For this review, take the finished solid that the model builds, in its own axes (mm). Coordinates: 2 decimals unless noted, no trailing zeros. Order: outer loops, then holes, each group sorted by start corner. A loop starts at its lowest first (then second) coordinate and runs counter-clockwise, first axis right, second up.
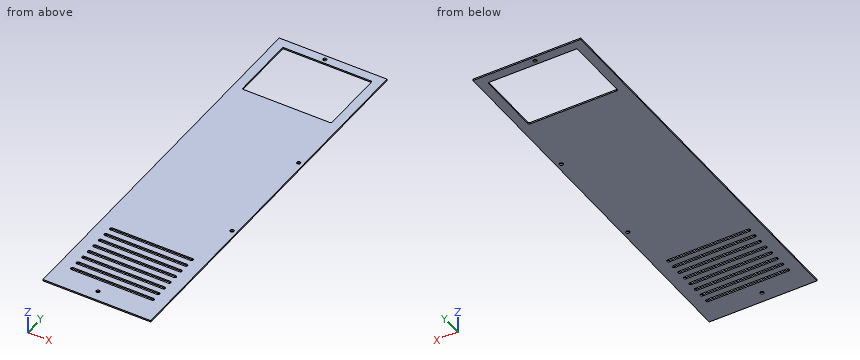
from build123d import *

# Parameters (mm, degrees)
SKETCH1_W           = 225.9076
SKETCH1_H           = 810.1076
BOSS_EXTRUDE1_DEPTH = 3.0734
VENTMASTER_DEPTH    = 421.519425968
LPATTERN1_COUNT     = 8
LPATTERN1_PITCH     = 19.05
CUT_EXTRUDE2_DEPTH  = 3.0734
SKETCH4_R           = 3.81
CUT_EXTRUDE3_DEPTH  = 421.519425968


# Read off the part's stored shape, not the designer's step: Cut-Extrude2
with BuildPart() as part:
    # Sketch1 → Boss-Extrude1 (new body)
    with BuildSketch(Plane.XY):
        Rectangle(SKETCH1_W, SKETCH1_H)
    extrude(amount=BOSS_EXTRUDE1_DEPTH)

    # Sketch2 → VentMaster (cut, through all)
    with BuildSketch(Plane.XY.offset(3.0734)):
        with BuildLine():
            Line((-84.3788, -347.9038), (83.9978, -347.9038))
            ThreePointArc((83.9978, -347.9038), (87.1728, -351.0788), (83.9978, -354.2538))
            Line((83.9978, -354.2538), (-84.3788, -354.2538))
            ThreePointArc((-84.3788, -354.2538), (-87.5538, -351.0788), (-84.3788, -347.9038))
        make_face()
    ventmaster = extrude(amount=-VENTMASTER_DEPTH, mode=Mode.SUBTRACT)

    # LPattern1: VentMaster ×8
    with Locations(*[(0, i * LPATTERN1_PITCH, 0) for i in range(1, LPATTERN1_COUNT)]):
        add(ventmaster, mode=Mode.SUBTRACT)

    # Cut-Extrude2 outline → Cut-Extrude2 (cut)
    with BuildSketch(Plane.XY):
        with BuildLine():
            Line((-93.5228, 383.0828), (-93.5228, 248.4628))
            ThreePointArc((-93.5228, 248.4628), (-92.778851224, 246.666748776), (-90.9828, 245.9228))
            Line((-90.9828, 245.9228), (90.9828, 245.9228))
            ThreePointArc((90.9828, 245.9228), (92.778851224, 246.666748776), (93.5228, 248.4628))
            Line((93.5228, 248.4628), (93.5228, 383.0828))
            ThreePointArc((93.5228, 383.0828), (92.778851224, 384.878851224), (90.9828, 385.6228))
            Line((90.9828, 385.6228), (-90.9828, 385.6228))
            ThreePointArc((-90.9828, 385.6228), (-92.778851224, 384.878851224), (-93.5228, 383.0828))
        make_face()
    extrude(amount=CUT_EXTRUDE2_DEPTH, mode=Mode.SUBTRACT)

    # Sketch4 → Cut-Extrude3 (cut, through all)
    with BuildSketch(Plane.XY.offset(3.0734)):
        with Locations((-11.2522, 395.1478)):
            Circle(SKETCH4_R)
        with Locations((-11.2522, -382.8288)):
            Circle(SKETCH4_R)
        with Locations((103.0478, -109.7026)):
            Circle(SKETCH4_R)
        with Locations((103.0478, 118.5418)):
            Circle(SKETCH4_R)
    extrude(amount=-CUT_EXTRUDE3_DEPTH, mode=Mode.SUBTRACT)


solid = part.part
1. Take a section at B-B, the plane x = -26.5. Give the number of separate pieces and of enclosed holes in the cut face, plus the area to 3 significant figures.
Answer below:
separate pieces: 10
enclosed holes: 0
area: 1,900 mm2
2. Take a section at A-A, the plane y = 341.5. Give the boundary of the cut face in (x, z), plus the area to 3 significant figures.
Answer below:
outline: (-112.95, 0) - (-93.52, 0) - (-93.52, 3.07) - (-112.95, 3.07) - close; (93.52, 0) - (112.95, 0) - (112.95, 3.07) - (93.52, 3.07) - close
area: 119 mm2
3. To check wall thickness, follow L1, parallel to X at y = 286.5, z = 1.9; L2, parallel to X at y = -106.5, z = 1.7. State the ranges of each line that lie inside material, in increasing order.
Answer below:
L1: x = -112.95 to -93.52, 93.52 to 112.95
L2: x = -112.95 to 100.98, 105.11 to 112.95
